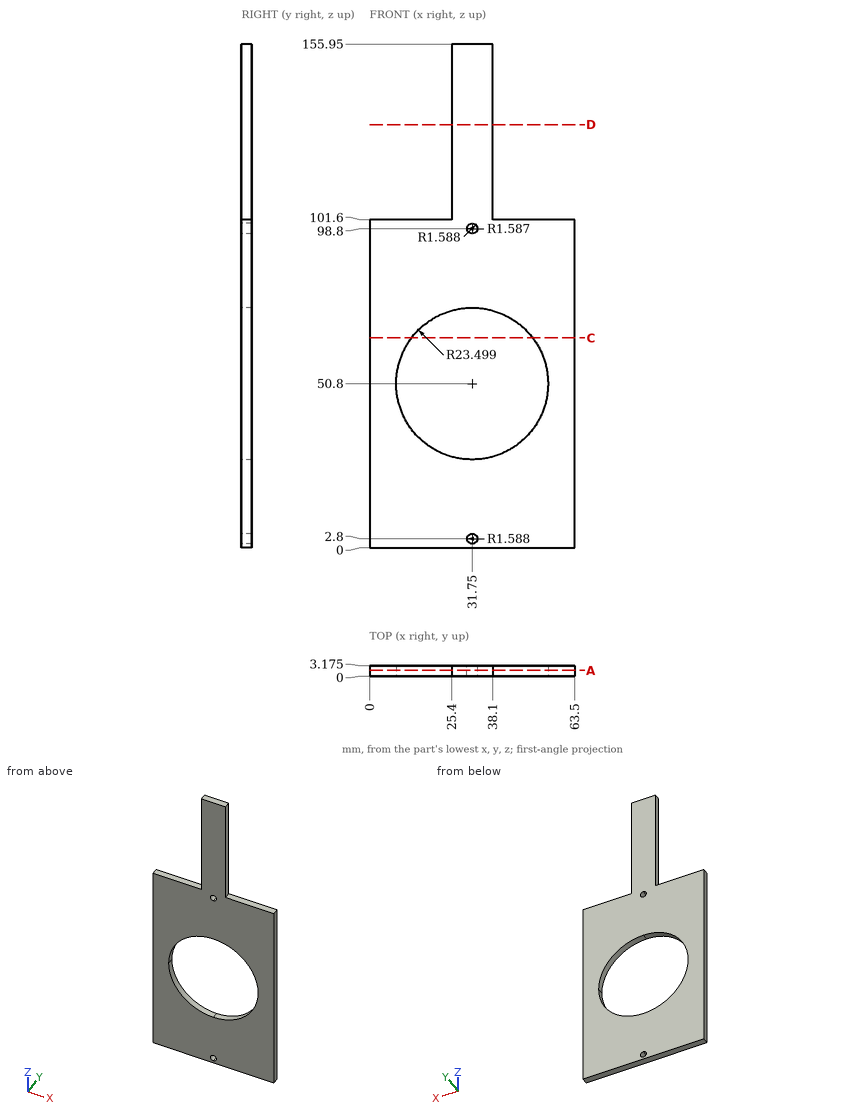
Could you check a few things on this drawing? It's one solid part, dimensions in mm from its lowest x, y, z. Coordinates: 2 decimals unless noted, no trailing zeros. Write each loop counter-clockwise with the first axis right and the second up, starting at its lowest first coordinate (ties: lowest second). Pieces come first, ordered by that corner, then holes.
Q1. Please list where these lines run through material, in increasing order: L1, parallel to Z at x = 31.5, y = 1.65; L2, parallel to Z at x = 7, y = 0.25; L3, parallel to X at y = 3.05, z = 120.
Results found:
L1: z = 0 to 1.23, 4.37 to 27.3, 74.3 to 97.23, 100.37 to 155.95
L2: z = 0 to 101.6
L3: x = 25.4 to 38.1
Q2. Imagine slicing it at A-A, the plane y = 1.75. Count the separate pieces of the cut face and the enclosed holes in it, plus the area to 3 significant figures.
Results found:
separate pieces: 1
enclosed holes: 3
area: 5,390 mm2
Q3. Imagine slicing it at D-D, the plane z = 131. List the corners of the cut face in (x, y) for me (1 decimal).
Results found:
outline: (25.4, 0) - (38.1, 0) - (38.1, 3.2) - (25.4, 3.2) - close
Q4. Imagine slicing it at C-C, the plane z = 65. List the corners of the cut face in (x, y) for me (1 decimal).
Results found:
outline: (0, 0) - (13, 0) - (13, 3.2) - (0, 3.2) - close; (50.5, 0) - (63.5, 0) - (63.5, 3.2) - (50.5, 3.2) - close
Q5. For P1, Ø1.6, axis at y = 1.5, z = 128, coming from the +X side; P2, Ø1.6, axis at x = 12.5, y = 1.5, coming from the +Z side, each with a flat end and sliding along its axis, tell me the tip position at first contact or that it passes through.
Results found:
P1: stops at x = 38.1
P2: stops at z = 101.6
